Verification items for this drawing (mm, ordinates from the low corner). Give positions to 0.01 mm unless a question says otherwise; leave off trailing zeros. Write each loop counter-clockwise with the first axis right and the second up, starting at its lowest first coordinate (ties: lowest second). Pieces come first, ordered by that corner, then holes. Notation, with made-up numbers: (76.25, 15) -> (129.25, 15) arc R18 ccw to (129.25, 41) -> close; hole circle Ø5 at (-3, -12). An arc over 180 degrees is marked (long way). Write item = value, one per line.
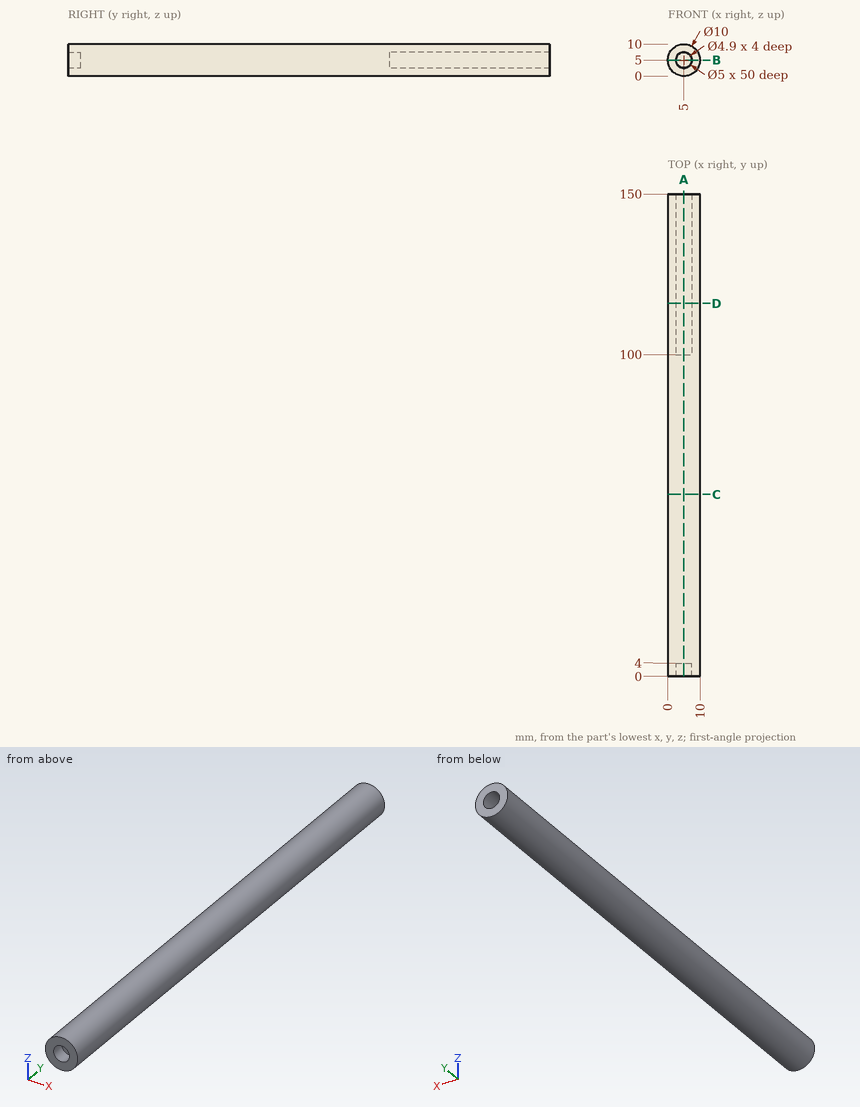
Item 1: Sectioned sample at A-A on x = 5. Record the cut outline in (y, z).
Response values:
outline = (0, 0) -> (150, 0) -> (150, 2.5) -> (100, 2.5) -> (100, 7.5) -> (150, 7.5) -> (150, 10) -> (0, 10) -> (0, 7.45) -> (4, 7.45) -> (4, 2.55) -> (0, 2.55) -> close
Item 2: Sectioned sample at B-B on z = 5. Record the cut outline in (x, y).
Response values:
outline = (0, 0) -> (2.55, 0) -> (2.55, 4) -> (7.45, 4) -> (7.45, 0) -> (10, 0) -> (10, 150) -> (7.5, 150) -> (7.5, 100) -> (2.5, 100) -> (2.5, 150) -> (0, 150) -> close
Item 3: Go/stop test with flat-tipped pins: P1, Ø5, axis at x = 7.5, y = 25, coming from the +Z side; P2, Ø3, axis at x = 5, z = 5, coming from the -Y side; P3, Ø4.5, axis at x = 5, z = 5, coming from the +Y side. Record where each tip stops, or that it passes through.
Response values:
P1 = 10
P2 = 4
P3 = 100
Item 4: Sectioned sample at D-D on y = 116. Record the cut outline in (x, z), then the cut area to 3 significant figures.
Response values:
outline = circle Ø10 at (5, 5); hole circle Ø5 at (5, 5)
area = 58.9 mm^2
Item 5: Sectioned sample at C-C on y = 56.5. Record the cut outline in (x, z).
Response values:
outline = circle Ø10 at (5, 5)
Item 6: Material ranges on line 1 (Z direction, x = 5, y = 125); line 2 (X direction, y = 2, z = 5), recorded low to high.
Response values:
line_1 = 0 to 2.5, 7.5 to 10
line_2 = 0 to 2.55, 7.45 to 10
